The figure shows three views and two pictorial views of one solid part (mm, origin at its lowest corner). Answer the questions. A direction names the side the tool comes from. Give positions to 0.01 mm unless a question says otherwise; leave off trailing zeros. Order: outer loops, then holes, each group sorted by start corner. A loop starts at its lowest first (then second) coordinate and runs counter-clockwise, first axis right, second up. Notation, with made-up numbers: (-8.5, -36) - (49.5, -36) arc R21 ccw to (49.5, -3) - close; hole circle Ø2 at (-37.5, 44). An arc over 180 degrees is marked (long way). Use a Markdown table: item, result. Add a question column.
1. For a pull along X with two mould halves and no side action, classify the marked faces 1, 2, 3 and 4 as released by +X, released by -X, zero draft, split by the parting line, or undercut.
2. Consider L1, parallel to Y at x = 6, z = 53.5; L2, parallel to X at y = 17.5, z = 18; L3, parallel to Y at x = 17, z = 52.5. Determine where each line is inside the solid, lowest interval first.
3. Flat-ended cylindrical pins translate along their axes: P1, Ø1, axis at y = 10, z = 38.5, coming from the +X side; P2, Ø1.9, axis at y = 25, z = 6.5, coming from the +X side; P3, Ø16, axis at y = 28.5, z = 14.5, coming from the -X side; P4, Ø3, axis at x = 32.5, y = 36.5, coming from the +Z side. Find the tip coordinate at first contact, or state that the pin passes through.
4. A cutting plane is placed at B-B on y = 8. Determine the outline of the cut face in (x, z).
5. A cutting plane is placed at D-D on z = 17. Determine the outline of the cut face in (x, y), and give its area (3 significant figures).
6. A cutting plane is placed at A-A on z = 53.5. Determine the outline of the cut face in (x, y), and give its area (3 significant figures).
7. Which of the six approach directions +Z, -Z, +X, -X, +Y, -Y give full straight-line access (tool end or side, diameter ignored) to the marked faces 5 and 6?
8. A cutting plane is placed at C-C on x = 8. Determine the outline of the cut face in (y, z).
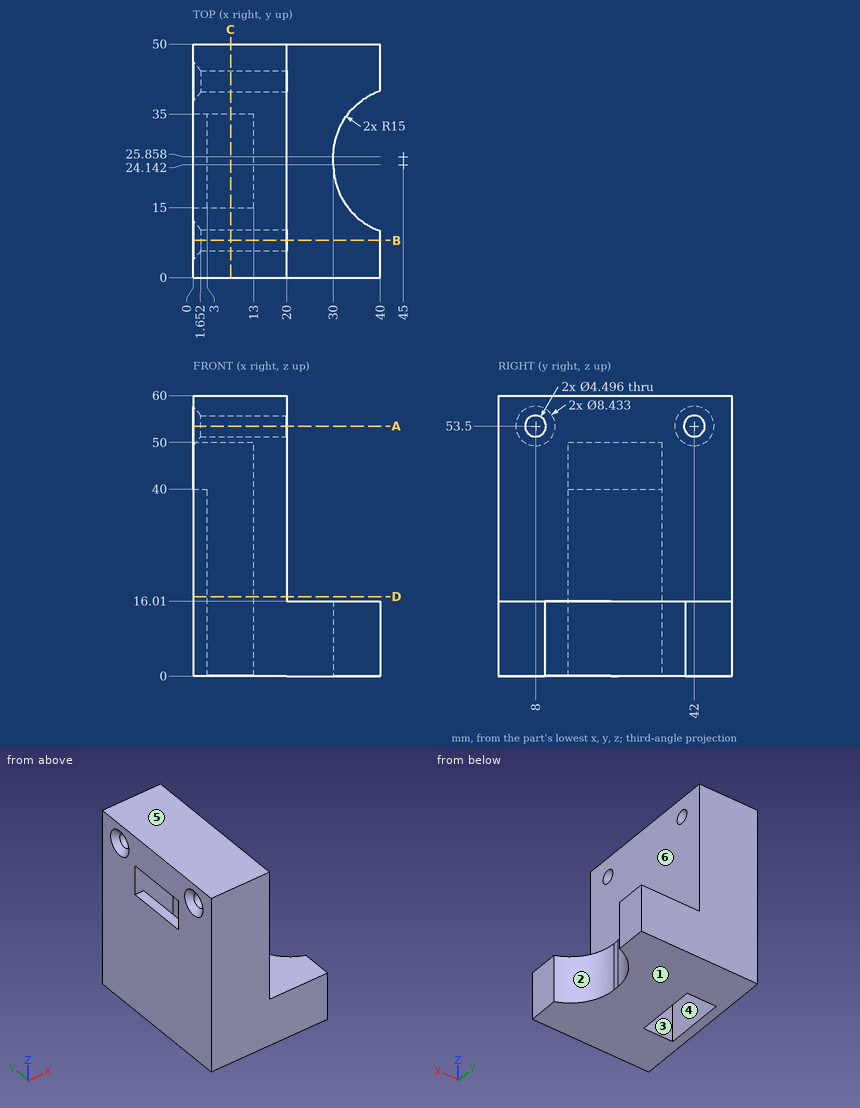
Output values:
| question | item | result |
|---|---|---|
| 1 | face 1 | zero draft |
| 1 | face 2 | released by +X |
| 1 | face 3 | undercut |
| 1 | face 4 | undercut |
| 2 | L1 | 0 to 5.75, 10.25 to 39.75, 44.25 to 50 |
| 2 | L2 | 0 to 3, 13 to 20 |
| 2 | L3 | 0 to 5.99, 10.01 to 39.99, 44.01 to 50 |
| 3 | P1 | x = 20 |
| 3 | P2 | x = 30 |
| 3 | P3 | x = 0 |
| 3 | P4 | z = 16.01 |
| 4 | outline | (0, 0) - (40, 0) - (40, 16.01) - (20, 16.01) - (20, 51.25) - (1.65, 51.25) - (0, 49.28) - close; (0, 57.72) - (1.65, 55.75) - (20, 55.75) - (20, 60) - (0, 60) - close |
| 5 | outline | (0, 0) - (20, 0) - (20, 50) - (0, 50) - close; hole (3, 15) - (13, 15) - (13, 35) - (3, 35) - close |
| 5 | area | 800 mm² |
| 6 | outline | (0, 0) - (20, 0) - (20, 5.75) - (1.65, 5.75) - (0, 3.78) - close; (0, 12.22) - (1.65, 10.25) - (20, 10.25) - (20, 39.75) - (1.65, 39.75) - (0, 37.78) - close; (0, 46.22) - (1.65, 44.25) - (20, 44.25) - (20, 50) - (0, 50) - close |
| 6 | area | 814 mm² |
| 7 | face 5 | +Z, +X, -X, +Y, -Y |
| 7 | face 6 | +Z, +X, +Y, -Y |
| 8 | outline | (0, 0) - (15, 0) - (15, 50) - (35, 50) - (35, 0) - (50, 0) - (50, 60) - (0, 60) - close; hole circle Ø4.5 at (8, 53.5); hole circle Ø4.5 at (42, 53.5) |
